Geometry: final body of the model. Coordinates: model frame, mm. A direction names the side the tool comes from. Give positions to 0.01 mm unless a question says otherwise; leave off trailing zeros. Write each loop counter-clockwise with the first axis right and the second up, starting at its lowest first coordinate (ties: lowest second). Pieces come first, ordered by that corner, then holes.
Q1. Cut plane B-B on x = 0. Return the cut outline in (y, z).
Q2. Cut plane A-A on z = 0. Return the cut outline in (x, y).
Q3. Line query: L1, parallel to Y at x = -0.5, z = 1.25; L2, parallel to X at y = 98, z = 4; L3, parallel to Z at x = 3, y = 83. Output: solid intervals per line, ascending.
Q4. Draft query along X for faces 3 (the face through (-4.88, 59.16, -1.08)), 4 (the face through (0, 0, 0)), 5 (the face through (3, 37, 0)). Return one class per face: pulls with the +X half, pulls with the -X half, needs draft (parallel to the pull), parting line crosses it, or undercut.
Q5. Cut plane C-C on y = 12. Return the cut outline in (x, z), plus the area to 3 significant figures.
Q6. Pin query (flat end, axial travel): pin 1 (3 mm diameter, centred on y = 52, z = 3.5, fed in from +X); pin 2 (1.5 mm diameter, centred on y = 76, z = 2, fed in from +X); pin 3 (1.2 mm diameter, centred on y = 37.5, z = -1.5, fed in from +X). Return the tip coordinate at first contact, or that it passes through.
Q7. Reachability of faces 1 (the face through (0, 39.032, 0)), 2 (the face through (0, 120, 0)) from +Z, -Z, +X, -X, +Y, -Y: full face, straight path, thin tool, end or side. Return the list, or none.
```python
from build123d import *

# Parameters (mm, degrees)
SKETCH1_R           = 5
BOSS_EXTRUDE1_DEPTH = 120
SKETCH2_W           = 6
SKETCH2_H           = 4
CUT_EXTRUDE1_DEPTH  = 60


with BuildPart() as part:
    # Sketch1 → Boss-Extrude1 (new body)
    with BuildSketch(Plane(origin=(0, 0, 0), x_dir=(1, 0, 0), z_dir=(0, 1, 0))):
        with Locations(Location((0, 0, 0), (0, 0, 270))):
            Circle(SKETCH1_R)
    extrude(amount=BOSS_EXTRUDE1_DEPTH)

    # Sketch2 → Cut-Extrude1 (cut, symmetric)
    with BuildSketch(Plane.XY):
        with Locations((0, 37.032253422)):
            Rectangle(SKETCH2_W, SKETCH2_H)
    extrude(amount=CUT_EXTRUDE1_DEPTH, both=True, mode=Mode.SUBTRACT)


solid = part.part
```
Data:
1. outline: (0, -5) - (35.03, -5) - (35.03, 5) - (0, 5) - close; (39.03, -5) - (120, -5) - (120, 5) - (39.03, 5) - close
2. outline: (-5, 0) - (5, 0) - (5, 120) - (-5, 120) - close; hole (-3, 35.03) - (3, 35.03) - (3, 39.03) - (-3, 39.03) - close
3. L1: y = 0 to 35.03, 39.03 to 120
3. L2: x = -3 to 3
3. L3: z = -4 to 4
4. face 3: parting line crosses it
4. face 4: needs draft
4. face 5: undercut
5. outline: circle Ø10 at (0, 0)
5. area: 78.5 mm2
6. pin 1: stops at x = 4.58
6. pin 2: stops at x = 4.84
6. pin 3: stops at x = 4.92
7. face 1: +Z, -Z
7. face 2: +Z, -Z, +X, -X, +Y
